Autodesk Inventor part; units mm, degrees
ref_plane "YZ Plane" through (0, 0, 0) normal (1, 0, 0) x (0, 1, 0)
ref_plane "XZ Plane" through (0, 0, 0) normal (0, 1, 0) x (-1, 0, 0)
ref_plane "XY Plane" through (0, 0, 0) normal (0, 0, 1) x (1, 0, 0)
sketch "Skizze1" plane through (0, 0, 0) normal (0, 0, 1) x (1, 0, 0)
  line L0 (-27.25, -38) -> (27.25, -38)
  line L1 (27.25, -38) -> (27.25, 38)
  line L2 (27.25, 38) -> (-27.25, 38)
  line L3 (-27.25, 38) -> (-27.25, -38)
  line L4 (-27.25, -38) -> (27.25, 38) construction
  line L5 (27.25, -38) -> (-27.25, 38) construction
  line L6 (-29.25, -40) -> (29.25, -40)
  line L7 (29.25, -40) -> (29.25, 40)
  line L8 (29.25, 40) -> (-29.25, 40)
  line L9 (-29.25, 40) -> (-29.25, -40)
  line L10 (-29.25, -40) -> (29.25, 40) construction
  line L11 (29.25, -40) -> (-29.25, 40) construction
  point P0 (0, 0)
  dimension "d0" = 54.5
  dimension "d1" = 76
  dimension "d2" = 2
  dimension "d3" = 2
extrude "Extrusion1" add sketch "Skizze1" against normal blind 2.5 contours L3 L2 L1 L0 | L9 L8 L7 L6
extrude "Extrusion2" add sketch "Skizze1" along normal blind 25
sketch "Skizze2" plane through (0, 0, 25) normal (0, 0, 1) x (1, 0, 0)
  line L0 (27.25, -38) -> (-27.25, -38)
  line L1 (27.25, 38) -> (27.25, -38)
  line L2 (29.25, -40) -> (29.25, 40)
  line L3 (29.25, 40) -> (-29.25, 40)
  line L4 (-27.25, 38) -> (27.25, 38)
  line L5 (-29.25, -40) -> (29.25, -40)
  line L6 (27.25, -38) -> (27.25, 38)
  line L7 (29.25, 40) -> (29.25, -40)
  line L8 (27.25, -38) -> (29.25, -38)
  line L9 (29.25, -38) -> (29.25, -17)
  line L10 (29.25, -17) -> (27.25, -17)
  line L11 (27.25, -17) -> (27.25, -38)
  point P0 (0, 0)
  dimension "d8" = 21
extrude "Extrusion3" cut sketch "Skizze2" against normal up to surface (25 mm away)
sketch "Skizze3" plane through (0, 0, 25) normal (0, 0, 1) x (1, 0, 0)
  line L0 (-27.25, 38) -> (27.25, 38)
  line L1 (29.25, 40) -> (-29.25, 40)
  line L2 (27.25, 38) -> (27.25, -17)
  line L3 (27.25, 38) -> (7.25, 38)
  line L4 (7.25, 38) -> (7.25, 40)
  line L5 (7.25, 40) -> (27.25, 40)
  line L6 (27.25, 40) -> (27.25, 38)
  point P0 (0, 0)
  dimension "d11" = 20
extrude "Extrusion4" cut sketch "Skizze3" against normal blind 15
chamfer "Fase1" distance 1.5 angle 45 4 edges at (28.25, -17, 0) (1, -38, 0) (7.25, 39, 10) (27.25, 39, 10)
sketch "Skizze4" plane through (0, 0, 25) normal (0, 0, 1) x (1, 0, 0)
  line L0 (-27.25, -38) -> (-27.25, 38)
  line L1 (29.25, -38) -> (-27.25, -38)
  line L2 (-29.25, -40) -> (29.25, -40)
  line L3 (-27.25, -38) -> (29.25, -38)
  line L4 (-27.25, -38) -> (-27.25, -40)
  line L5 (29.25, -40) -> (-29.25, -40)
  line L6 (-27.25, -40) -> (-15.5394, -40)
  line L7 (-15.5394, -38) -> (-15.5394, -40)
  line L8 (-15.5394, -38) -> (-27.25, -38)
  point P0 (0, 0)
  dimension "d17" = 11.7106
extrude "Extrusion5" cut sketch "Skizze4" against normal blind 5
equation "\"d3\" = d2"
properties part number "housing-lvl-bottom" material "ABS-Kunststoff"
Input: part model. Units: mm. Frame: model coordinates. A direction names the side the tool comes from. Coordinates: 2 decimals unless noted, no trailing zeros. Loops run counter-clockwise (first coordinate to the right, second up) from the corner with the lowest first, then second, coordinate; pieces in that order, holes last.
(1) Section C-C on x = -2. Return the cut outline in (y, z).
(2) Material intervals for probe 1 along X at (y, z) = (9.5, 21); probe 2 along Y at (x, z) = (1, 10.5); probe 3 along Z at (x, y) = (7, -22.5), sorted ascending.
(3) Section D-D on z = 5.25. Return the cut outline in (x, y), then the cut area to 3 significant figures.
(4) Pull-direction query (X, two-part tool) for faces 6 (the face through (1, -38, 13)), 7 (the face through (-29.25, 1, 11)), 8 (the face through (-21, -39, 20)); classes: released by +X, released by -X, zero draft, split by the parting line, or undercut.
(5) First-contact query: pin 1 Ø1 at (x, y) = (-19.5, -39) entering from +Z; pin 2 Ø1.6 at (x, y) = (15.5, 38.5) entering from +Z; pin 3 Ø5 at (x, y) = (23, -8.5) entering from +Z. Flat tips, straight axial feed; report the tip coordinate or a pass-through.
(6) Section A-A on z = 15.5. Return the cut outline in (x, y).
(7) Set-up query: faces 1 (the face through (-15.539, -39, 23)), 2 (the face through (28, -17, 13)), 3 (the face through (17, 39, 10)), 4 (the face through (-6, 38, 12)), 5 (the face through (29.25, 8, 11)). Return all of +Z, -Z, +X, -X, +Y, -Y with unobstructed straight access to the full face (end or side cutting, diameter ignored); none if empty.
(8) Section B-B on z = 22.5. Return the cut outline in (x, y), then the cut area to 3 significant figures.
Data:
1. outline: (-40, -2.5) - (40, -2.5) - (40, 25) - (38, 25) - (38, 0) - (-36.5, 0) - (-38, 1.5) - (-38, 25) - (-40, 25) - close
2. probe 1: x = -29.25 to -27.25, 27.25 to 29.25
2. probe 2: y = -40 to -38, 38 to 40
2. probe 3: z = -2.5 to 0
3. outline: (-29.25, -40) - (29.25, -40) - (29.25, -38) - (-27.25, -38) - (-27.25, 38) - (27.25, 38) - (27.25, -17) - (29.25, -17) - (29.25, 40) - (-29.25, 40) - close
3. area: 496 mm2
4. face 6: zero draft
4. face 7: released by -X
4. face 8: undercut
5. pin 1: stops at z = 20
5. pin 2: stops at z = 10
5. pin 3: stops at z = 0
6. outline: (-29.25, -40) - (29.25, -40) - (29.25, -38) - (-27.25, -38) - (-27.25, 38) - (7.25, 38) - (7.25, 40) - (-29.25, 40) - close; (27.25, -17) - (29.25, -17) - (29.25, 40) - (27.25, 40) - close
7. face 1: +Z, -Y
7. face 2: +Z, +X
7. face 3: +Z, +Y
7. face 4: +Z
7. face 5: +Z, -Z, +X, +Y, -Y
8. outline: (-29.25, -40) - (-27.25, -40) - (-27.25, 38) - (7.25, 38) - (7.25, 40) - (-29.25, 40) - close; (-15.54, -40) - (29.25, -40) - (29.25, -38) - (-15.54, -38) - close; (27.25, -17) - (29.25, -17) - (29.25, 40) - (27.25, 40) - close
8. area: 433 mm2
